Verification items for this drawing (mm, ordinates from the low corner). Round coordinates to 2 decimals unless told otherwise and drop trailing zeros. Loops run counter-clockwise (first coordinate to the right, second up) from the corner with the lowest first, then second, coordinate; pieces in that order, holes last. Notation, with made-up numbers: (46.25, 29.5) - (99.25, 29.5) arc R12 cw to (99.25, 41.5) - close; hole circle Ø3 at (-6.75, 10.25). An arc over 180 degrees is marked (long way). Use a Markdown table: item, result. Add a question column.
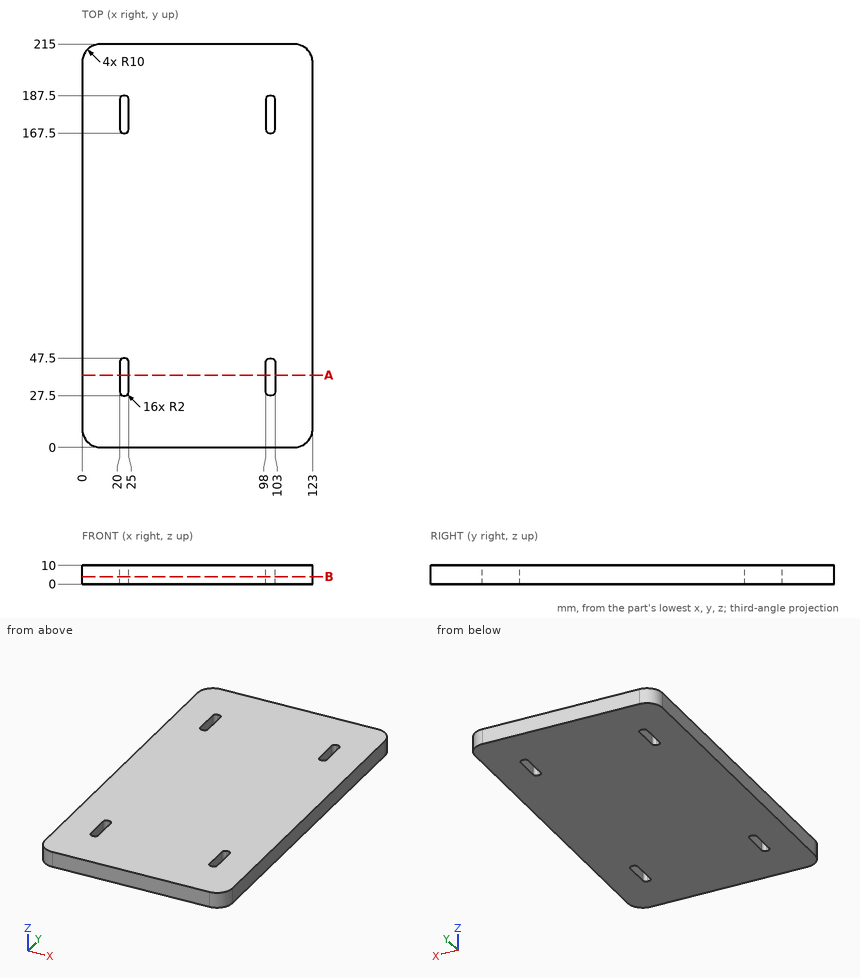
Q1. Go/stop test with a flat-tipped pin: pin 1 Ø0.8 at (x, z) = (22.5, 4.5) entering from -Y. Record where the tip stops, or that it passes through.
Q2. Thickness scan on line 1 along X through (y, z) = (39.5, 1). Record the ranges inside material, lowest first.
Q3. Section check A-A on y = 38.5. Record the cut outline in (x, z).
Q4. Section check B-B on z = 4. State how many separate pieces and enclosed holes the cut face has, plus the area to 3 significant figures.
Determined:
| question | item | result |
|---|---|---|
| 1 | pin 1 | stops at y = 0 |
| 2 | line 1 | x = 0 to 20, 25 to 98, 103 to 123 |
| 3 | outline | (0, 0) - (20, 0) - (20, 10) - (0, 10) - close; (25, 0) - (98, 0) - (98, 10) - (25, 10) - close; (103, 0) - (123, 0) - (123, 10) - (103, 10) - close |
| 4 | separate pieces | 1 |
| 4 | enclosed holes | 4 |
| 4 | area | 26,000 mm² |
